```python
from build123d import *

# Parameters (mm, degrees)
SM_BASE_FLANGE_1_DEPTH = 1.5


# Sheet-metal steps are written as plain solids
with BuildPart() as part:
    # Sketch 1 → Базовая кромка1 (new body)
    with BuildSketch(Plane(origin=(0, 0, 0), x_dir=(0, 0, -1), z_dir=(1, 0, 0))):
        with BuildLine():
            Line((0, 0), (10.5, 0))
            ThreePointArc((10.5, 0), (10.758819045, -0.034074174), (11, -0.133974596))
            Line((11, -0.133974596), (69, -33.620290209))
            ThreePointArc((69, -33.620290209), (70, -33.620290209), (70.5, -32.754264805))
            Line((70.5, -32.754264805), (70.5, 40.70428331))
            ThreePointArc((70.5, 40.70428331), (70.366025404, 41.20428331), (70, 41.570308714))
            Line((70, 41.570308714), (9.964101615, 76.232050808))
            ThreePointArc((9.964101615, 76.232050808), (9.481739705, 76.431851653), (8.964101615, 76.5))
            Line((8.964101615, 76.5), (0, 76.5))
            Line((0, 76.5), (0, 0))
        make_face()
    extrude(amount=-SM_BASE_FLANGE_1_DEPTH)


solid = part.part
```
Source: CAD feature listing. Evaluate the final solid. Frame: model axes, mm. Give positions to 0.01 mm unless a question says otherwise; leave off trailing zeros. Order: outer loops, then holes, each group sorted by start corner. A loop starts at its lowest first (then second) coordinate and runs counter-clockwise, first axis right, second up.
(1) Material intervals for line 1 along Y through (x, z) = (-0.15, -60.5); line 2 along Y through (x, z) = (-0.15, -23); line 3 along Z through (x, y) = (-0.75, 42), sorted ascending.
(2) Section query A-A (x = -0.8). Return the cut outline in (y, z).
(3) Section query B-B (z = -3.5). Return the cut outline in (x, y).
(4) Contact query for a flat-ended pin moving along its axis: P1, Ø0.8, axis at x = -0.5, z = -3, coming from the -Y side. Output: stop coordinate, or through.
(5) Pull-direction query (Y, two-part tool) for faces 1 (the face through (-0.74, -16.64, -39.59)), 2 (the face through (-1.5, 22, -35)), 3 (the face through (-0.74, 58.66, -40.4)); classes: +Y half, -Y half, draft (parallel to the pull), parting line (faces both ways), or undercut.
(6) Section query C-C (y = 64.5). Return the cut outline in (x, z), plus the area to 3 significant figures.
Outcome:
1. line 1: y = -28.71 to 47.06
1. line 2: y = -7.06 to 68.71
1. line 3: z = -69.26 to 0
2. outline: (-33.62, -69) arc R1 ccw to (-32.75, -70.5) - (40.7, -70.5) arc R1 ccw to (41.57, -70) - (76.23, -9.96) arc R2 ccw to (76.5, -8.96) - (76.5, 0) - (0, 0) - (0, -10.5) arc R1 cw to (-0.13, -11) - close
3. outline: (-1.5, 0) - (0, 0) - (0, 76.5) - (-1.5, 76.5) - close
4. P1: stops at y = 0
5. face 1: -Y half
5. face 2: draft
5. face 3: +Y half
6. outline: (-1.5, -30.28) - (0, -30.28) - (0, 0) - (-1.5, 0) - close
6. area: 45.4 mm2
